For this review, take the finished solid that the model builds, in its own axes (mm). Face numbers are marked on the shaded views. A direction names the side the tool comes from. Round coordinates to 2 decimals unless told otherwise and drop trailing zeros. Order: outer loops, then holes, each group sorted by start corner. A loop starts at its lowest first (then second) coordinate and runs counter-clockwise, first axis right, second up. Notation, with made-up numbers: M 76,-18 L 98,-18 A6 ccw 98,-7 Z; hole C 7.25,51.25 d8. An arc over 180 degrees is marked long. Put each result on its own line as item: value.
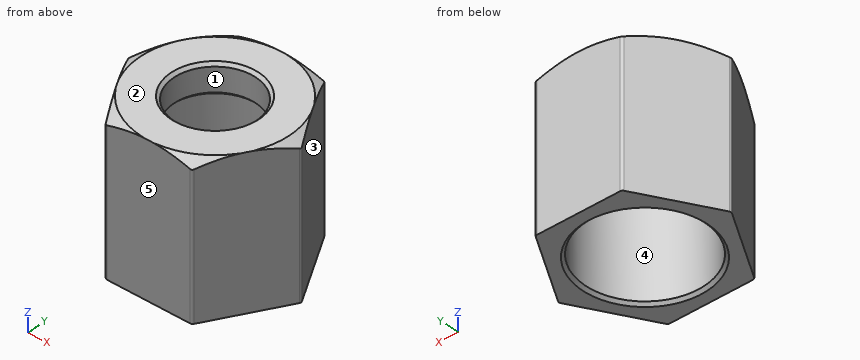
from build123d import *

# Parameters (mm, degrees)
ESTRUSIONE_ESTRUSIONE1_DEPTH = 10
SCHIZZO6_OUTSIDE_W           = 18.864
SCHIZZO6_OUTSIDE_H           = 17.316
SCHIZZO6_OUTSIDE_R           = 5
TAGLIO_ESTRUSIONE1_DEPTH     = 0.5
TAGLIO_ESTRUSIONE1_TAPER     = 59
RACCORDO1_R                  = 0.2
SCHIZZO19_R                  = 4
TAGLIO_ESTRUSIONE5_DEPTH     = 8
TAGLIO_ESTRUSIONE6_REACH     = 4
SCHIZZO20_R                  = 2.75
SMUSSO3_SIZE                 = 0.2


with BuildPart() as part:
    # Schizzo4 → Estrusione-Estrusione1 (new body)
    with BuildSketch(Plane.XY):
        Polygon((2.886751346, 5), (-2.886751346, 5), (-5.773502692, 0), (-2.886751346, -5), (2.886751346, -5), (5.773502692, 0), align=None)
    extrude(amount=-ESTRUSIONE_ESTRUSIONE1_DEPTH)

    # Schizzo6 outside → Taglio-Estrusione1 (cut)
    with BuildSketch(Plane.XY):
        Rectangle(SCHIZZO6_OUTSIDE_W, SCHIZZO6_OUTSIDE_H)
        Circle(SCHIZZO6_OUTSIDE_R, mode=Mode.SUBTRACT)
    extrude(amount=-TAGLIO_ESTRUSIONE1_DEPTH, taper=TAGLIO_ESTRUSIONE1_TAPER, mode=Mode.SUBTRACT)

    # Raccordo1
    raccordo1_edges = [part.edges().sort_by_distance(p)[0] for p in [
        (2.886751346, -5, -5.232383653),
        (-2.886751346, -5, -5.232383653),
        (-5.773502692, 0, -5.232383653),
        (-2.886751346, 5, -5.232383653),
        (2.886751346, 5, -5.232383653),
        (5.773502692, 0, -5.232383653),
    ]]
    fillet(raccordo1_edges, radius=RACCORDO1_R)

    # Schizzo19 → Taglio-Estrusione5 (cut)
    with BuildSketch(Plane(origin=(0, 0, -10), x_dir=(-1, 0, 0), z_dir=(0, 0, -1))):
        Circle(SCHIZZO19_R)
    extrude(amount=-TAGLIO_ESTRUSIONE5_DEPTH, mode=Mode.SUBTRACT)

    # Schizzo20 → Taglio-Estrusione6 (cut, up to next)
    with BuildSketch(Plane(origin=(0, 0, -2), x_dir=(-1, 0, 0), z_dir=(0, 0, -1)), mode=Mode.PRIVATE) as taglio_estrusione6_sk1:
        Circle(SCHIZZO20_R)
    taglio_estrusione6_tool1 = extrude(taglio_estrusione6_sk1.sketch, amount=-TAGLIO_ESTRUSIONE6_REACH, mode=Mode.PRIVATE) & part.part
    add(taglio_estrusione6_tool1.solids().sort_by_distance((0, 0, -2))[0], mode=Mode.SUBTRACT)

    # Smusso3
    smusso3_edges = [part.edges().sort_by_distance(p)[0] for p in [
        (4, 0, -10),
        (2.75, 0, 0),
        (2.75, 0, -2),
    ]]
    chamfer(smusso3_edges, length=SMUSSO3_SIZE)


solid = part.part
(1) For the marked faces 4 and 5, list the 3-axis set-ups (+Z, -Z, +X, -X, +Y, -Y) from which the entire face can be reached by the end or side of a thin tool; tool diameter is ignored.
A:
face 4: -Z
face 5: +Z, -Z, +X, -X, -Y
(2) To check wall thickness, follow L1, parallel to Y at x = 0, z = -2.75; L2, parallel to Y at x = 0, z = -1; L3, parallel to X at y = 2.25, z = -1.5. State the ranges of each line that lie inside material, in increasing order.
A:
L1: y = -5 to -4, 4 to 5
L2: y = -5 to -2.75, 2.75 to 5
L3: x = -4.47 to -1.58, 1.58 to 4.47
(3) Add section B-B on z = -7.25. Give the boundary of the cut face in (x, y), then the cut area to 3 significant figures.
A:
outline: M -5.72,-0.1 L -2.94,-4.9 A0.2 ccw -2.77,-5 L 2.77,-5 A0.2 ccw 2.94,-4.9 L 5.72,-0.1 A0.2 ccw 5.72,0.1 L 2.94,4.9 A0.2 ccw 2.77,5 L -2.77,5 A0.2 ccw -2.94,4.9 L -5.72,0.1 A0.2 ccw Z; hole C 0,0 d8
area: 36.3 mm2
(4) Add section A-A on z = -1. Give the boundary of the cut face in (x, y).
A:
outline: M -5.72,-0.1 L -2.94,-4.9 A0.2 ccw -2.77,-5 L 2.77,-5 A0.2 ccw 2.94,-4.9 L 5.72,-0.1 A0.2 ccw 5.72,0.1 L 2.94,4.9 A0.2 ccw 2.77,5 L -2.77,5 A0.2 ccw -2.94,4.9 L -5.72,0.1 A0.2 ccw Z; hole C 0,0 d5.5
(5) Insertion check: pin 1 Ø2 at (x, y) = (1.5, -2) entering from -Z; pin 2 Ø2.5 at (x, y) = (0.5, 1.5) entering from -Z; pin 3 Ø1 at (y, z) = (2.5, -5) entering from +X. Each pin has a flat end and moves straight along its axis. Give the tip position at first contact, or say it passes through.
A:
pin 1: stops at z = -2
pin 2: stops at z = -1.88
pin 3: stops at x = 4.62
(6) Draft analysis for pull direction X (two halves, no side actions). For the marked faces 1, 2 and 3, state which applies: released by +X, released by -X, zero draft, split by the parting line, or undercut.
A:
face 1: undercut
face 2: zero draft
face 3: released by +X
